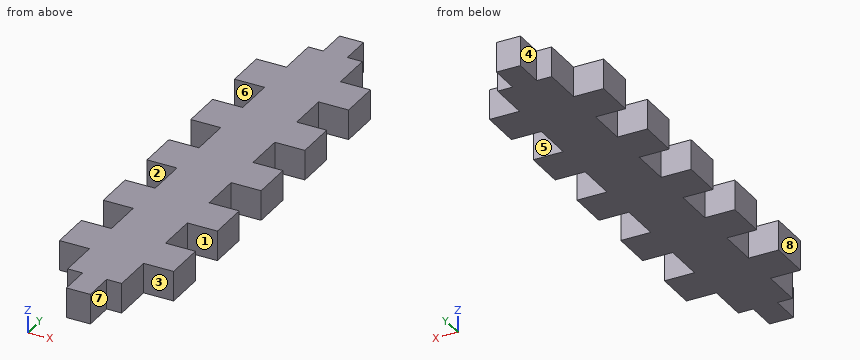
Autodesk Fusion 360 part; units mm, degrees
sketch "Sketch1" plane through (0, 0, 0) normal (0, 0, 1) x (1, 0, 0)
  line L0 (0, 0) -> (9, 0)
  line L1 (9, 0) -> (9, 74)
  line L2 (9, 74) -> (0, 74)
  line L3 (0, 74) -> (0, 0)
  dimension "d5" = 9
  dimension "d6" = 74
extrude "Extrude1" add sketch "Sketch1" along normal blind 5
sketch "Sketch2" plane through (9, 0, 0) normal (1, 0, 0) x (0, 1, 0)
  line L0 (0, 0) -> (74, 0)
  line L1 (74, 0) -> (74, 5)
  line L2 (74, 5) -> (0, 5)
  line L3 (0, 5) -> (0, 0)
  line L4 (6.7273, 5) -> (13.4545, 5)
  line L5 (13.4545, 5) -> (13.4545, 0)
  line L6 (13.4545, 0) -> (6.7273, 0)
  line L7 (6.7273, 0) -> (6.7273, 5)
  line L8 (20.1818, 0) -> (20.1818, 5)
  line L9 (20.1818, 5) -> (26.9091, 5)
  line L10 (26.9091, 5) -> (26.9091, 0)
  line L11 (26.9091, 0) -> (20.1818, 0)
  line L12 (33.6364, 0) -> (33.6364, 5)
  line L13 (33.6364, 5) -> (40.3636, 5)
  line L14 (40.3636, 5) -> (40.3636, 0)
  line L15 (40.3636, 0) -> (33.6364, 0)
  line L16 (47.0909, 0) -> (47.0909, 5)
  line L17 (47.0909, 5) -> (53.8182, 5)
  line L18 (53.8182, 5) -> (53.8182, 0)
  line L19 (53.8182, 0) -> (47.0909, 0)
  line L20 (60.5455, 0) -> (60.5455, 5)
  line L21 (60.5455, 5) -> (67.2727, 5)
  line L22 (67.2727, 5) -> (67.2727, 0)
  line L23 (67.2727, 0) -> (60.5455, 0)
  dimension "d9" = 6.7273
  dimension "d10" = 6.7273
  dimension "d13" = 53.8182
  dimension "d14" = 0
extrude "Extrude2" add sketch "Sketch2" along normal blind 5 contours L0 L2 L4 L5 L6 L7 | L0 L2 L8 L9 L10 L11 | L0 L2 L12 L13 L14 L15 | L0 L2 L16 L17 L18 L19 | L0 L2 L20 L21 L22 L23
sketch "Sketch3" plane through (0, 0, 0) normal (-1, 0, 0) x (0, -1, 0)
  line L0 (-74, 0) -> (0, 0)
  line L1 (0, 0) -> (0, 5)
  line L2 (0, 5) -> (-74, 5)
  line L3 (-74, 5) -> (-74, 0)
  line L4 (-67.2727, 5) -> (-60.5455, 5)
  line L5 (-60.5455, 5) -> (-60.5455, 0)
  line L6 (-60.5455, 0) -> (-67.2727, 0)
  line L7 (-67.2727, 0) -> (-67.2727, 5)
  line L8 (-53.8182, 0) -> (-53.8182, 5)
  line L9 (-53.8182, 5) -> (-47.0909, 5)
  line L10 (-47.0909, 5) -> (-47.0909, 0)
  line L11 (-47.0909, 0) -> (-53.8182, 0)
  line L12 (-40.3636, 0) -> (-40.3636, 5)
  line L13 (-40.3636, 5) -> (-33.6364, 5)
  line L14 (-33.6364, 5) -> (-33.6364, 0)
  line L15 (-33.6364, 0) -> (-40.3636, 0)
  line L16 (-26.9091, 0) -> (-26.9091, 5)
  line L17 (-26.9091, 5) -> (-20.1818, 5)
  line L18 (-20.1818, 5) -> (-20.1818, 0)
  line L19 (-20.1818, 0) -> (-26.9091, 0)
  line L20 (-13.4545, 0) -> (-13.4545, 5)
  line L21 (-13.4545, 5) -> (-6.7273, 5)
  line L22 (-6.7273, 5) -> (-6.7273, 0)
  line L23 (-6.7273, 0) -> (-13.4545, 0)
  dimension "d17" = 6.7273
  dimension "d18" = 6.7273
  dimension "d21" = 53.8182
  dimension "d22" = 0
extrude "Extrude3" add sketch "Sketch3" along normal blind 5 contours L0 L2 L4 L5 L6 L7 | L0 L2 L8 L9 L10 L11 | L0 L2 L12 L13 L14 L15 | L0 L2 L16 L17 L18 L19 | L0 L2 L20 L21 L22 L23
sketch "Sketch4" plane through (0, 0, 0) normal (0, 0, 1) x (1, 0, 0)
  line L0 (2.5, 0) -> (6.5, 0)
  line L1 (6.5, 0) -> (6.5, -5)
  line L2 (6.5, -5) -> (2.5, -5)
  line L3 (2.5, -5) -> (2.5, 0)
  line L4 (0, 0) -> (9, 0)
  line L5 (6.5, 0) -> (9, 0) construction
  line L6 (0, 0) -> (2.5, 0) construction
  line L7 (2.5, 74) -> (6.5, 74)
  line L8 (6.5, 74) -> (6.5, 79)
  line L9 (6.5, 79) -> (2.5, 79)
  line L10 (2.5, 79) -> (2.5, 74)
  line L11 (9, 74) -> (0, 74)
  line L12 (6.5, 74) -> (9, 74) construction
  line L13 (2.5, 74) -> (0, 74) construction
  dimension "d25" = 5
  dimension "d26" = 4
  dimension "d27" = 4
  dimension "d28" = 5
extrude "Extrude4" add sketch "Sketch4" along normal blind 5
equation "laius = 74 mm"
equation "korgus = 9 mm"
equation "laius_tapp = laius / 11"
equation "paksus = 5 mm"
equation "d5 = korgus"
equation "d6 = laius"
equation "d7 = paksus"
equation "d9 = laius_tapp"
equation "d10 = laius_tapp"
equation "d13 = laius - 3 * laius_tapp"
equation "d15 = paksus"
equation "d17 = laius_tapp"
equation "d18 = laius_tapp"
equation "d21 = laius - 3 * laius_tapp"
equation "d23 = paksus"
equation "d25 = paksus"
equation "d28 = paksus"
equation "d29 = paksus"
Geometry check sheet. Reference: the model listing, model coordinates, mm. Face numbers are marked on the shaded views. A direction names the side the tool comes from. Coordinates: 2 decimals unless noted, no trailing zeros. Order: outer loops, then holes, each group sorted by start corner. A loop starts at its lowest first (then second) coordinate and runs counter-clockwise, first axis right, second up. Notation, with made-up numbers: (11.5, -7.5) - (37.5, -7.5) arc R19 cw to (37.5, 17.5) - close; hole circle Ø6 at (-12.5, 54). An arc over 180 degrees is marked (long way). Answer in a Markdown table with one row per item. Add a question column.
1. Access from +Z, -Z, +X, -X, +Y, -Y to the whole of each face (thin tool, end or side, straight path). Record for the marked faces 5, 6, 7 and 8.
2. Section check C-C (x = 0.75). Enter the section's corners in (y, z).
3. Section check A-A (x = 12). Enter the section's corners in (y, z), plus the area to 3 significant figures.
4. Draft check along Y on the marked faces 1, 2, 3 and 4. Enter one of: +Y half, -Y half, draft (parallel to the pull), parting line (faces both ways), or undercut.
5. Section check B-B (y = 72). Enter the section's corners in (x, z).
6. Gauge pin test, flat ends, axial feed: pin 1 Ø2.5 at (x, z) = (-3.5, 2.5) entering from +Y; pin 2 Ø2.5 at (x, z) = (-1.5, 3.5) entering from -Y; pin 3 Ø1.2 at (x, z) = (1, 2) entering from -Y. Record the tip position at first contact, or that the pin passes through.
7. Material ranges on L1, parallel to Y at x = 12.25, z = 2; L2, parallel to X at y = 75.5, z = 1.45; L3, parallel to X at y = 4, z = 0.7, recorded low to high. Write a range as [from, to].
Data:
| question | item | result |
|---|---|---|
| 1 | face 5 | +Z, -Z, +X |
| 1 | face 6 | +Z, -Z, -X |
| 1 | face 7 | +Z, -Z, +X, -Y |
| 1 | face 8 | +Z, -Z, -X, +Y, -Y |
| 2 | outline | (0, 0) - (74, 0) - (74, 5) - (0, 5) - close |
| 3 | outline | (6.73, 0) - (13.45, 0) - (13.45, 5) - (6.73, 5) - close; (20.18, 0) - (26.91, 0) - (26.91, 5) - (20.18, 5) - close; (33.64, 0) - (40.36, 0) - (40.36, 5) - (33.64, 5) - close; (47.09, 0) - (53.82, 0) - (53.82, 5) - (47.09, 5) - close; (60.55, 0) - (67.27, 0) - (67.27, 5) - (60.55, 5) - close |
| 3 | area | 168 mm² |
| 4 | face 1 | undercut |
| 4 | face 2 | undercut |
| 4 | face 3 | -Y half |
| 4 | face 4 | draft |
| 5 | outline | (0, 0) - (9, 0) - (9, 5) - (0, 5) - close |
| 6 | pin 1 | stops at y = 67.27 |
| 6 | pin 2 | stops at y = 6.73 |
| 6 | pin 3 | stops at y = 0 |
| 7 | L1 | y = [6.73, 13.45], [20.18, 26.91], [33.64, 40.36], [47.09, 53.82], [60.55, 67.27] |
| 7 | L2 | x = [2.5, 6.5] |
| 7 | L3 | x = [0, 9] |
